CAD build for the part. Positions are in the model's coordinates, mm. A direction names the side the tool comes from. Give positions to 0.01 mm unless a question says otherwise; leave off trailing zeros. Order: outer loops, then holes, each group sorted by start corner. A loop starts at its lowest first (then second) coordinate and runs counter-clockwise, first axis right, second up. Notation, with made-up numbers: (37, 22.5) -> (79, 22.5) arc R23 ccw to (79, 34.5) -> close; hole circle Ø1 at (88, 28.5). An arc over 180 degrees is marked (long way). Use one line per item in the form item = value. Start each with the question number.
1) Mould opens along X. For faces 4 (the face through (-16.345, 29.521, 1.521)), 5 (the face through (-0.47, 58.4, -4.14)), 6 (the face through (-18.93, -43.5, 1.48)) say: pulls with the +X half, pulls with the -X half, needs draft (parallel to the pull), parting line crosses it, or undercut.
2) Probe line 1 (X direction, y = -25, z = 1.2); line 2 (Z direction, x = 15.5, y = 42); line 3 (Y direction, x = 0, z = 2.3). List the from-to ranges inside material, lowest first.
3) Cut at B-B, the plane x = -4. Give the cut face in (y, z).
4) Cut at D-D, the plane y = -14.5. Give the cut face in (x, z).
5) Tool access for faces 1 (the face through (15, 26, 2)), 2 (the face through (-20, 15, 0)), 3 (the face through (-17.5, 2, 2)): list every direction of +Z, -Z, +X, -X, +Y, -Y with a clear straight run to the whole face (end or side of a thin tool).
6) Cut at A-A, the plane y = 3. Give the cut face in (x, z).
7) Cut at C-C, the plane y = -27.5. Give the cut face in (x, z).
8) Drop flat-ended pins along their axis: P1, Ø2.5, axis at x = -14.5, z = -2.5, coming from the -Y side; P2, Ø1.5, axis at y = -29, z = 2, coming from the -X side; P3, Ø3, axis at x = -17.5, y = 30, coming from the -Z side; P4, Ø2.5, axis at x = -36, y = -40, coming from the +Z side. Give the stop position or say it passes through.
from build123d import *

# Parameters (mm, degrees)
SKETCH_1_R                  = 1.6
EXTRUDE_1_DEPTH             = 3
CUT_EXTRUDE_1_REACH         = 72.365
SKETCH_2_W                  = 30
SKETCH_2_H                  = 35
CUT_EXTRUDE_2_REACH         = 72.365
SKETCH_3_W                  = 35
SKETCH_3_H                  = 55
CUT_EXTRUDE_3_REACH         = 72.365
SKETCH_4_W                  = 25
SKETCH_4_H                  = 10
EXTRUDE_2_REACH             = 72.365
EXTRUDE_2_DIRECTION_2_REACH = 72.365
EXTRUDE_3_DEPTH             = 35
EXTRUDE_3_DEPTH_BACK        = 35
FILLET_1_R                  = 5
CUT_EXTRUDE_5_REACH         = 99.66
SKETCH_8_W                  = 70
SKETCH_8_H                  = 5
CUT_EXTRUDE_4_REACH         = 99.66
CUT_EXTRUDE_6_REACH         = 101.977
SKETCH_9_W                  = 30
SKETCH_9_H                  = 3
FILLET_2_R                  = 5
CUT_EXTRUDE_7_REACH         = 76.866
SKETCH_10_R                 = 1.25
SKETCH_11_R                 = 5
SKETCH_11_R_2               = 1.25
EXTRUDE_4_DEPTH             = 3


with BuildPart() as part:
    # 草图1 → 凸台-拉伸1 (new body)
    with BuildSketch(Plane.XY):
        Polygon((-30, 56), (30, 56), (42.5, -45), (-42.5, -45), align=None)
        with Locations((-32.5, 0)):
            Circle(SKETCH_1_R, mode=Mode.SUBTRACT)
        with Locations((32.5, 0)):
            Circle(SKETCH_1_R, mode=Mode.SUBTRACT)
        with Locations((-22, 44.5)):
            Circle(SKETCH_1_R, mode=Mode.SUBTRACT)
        with Locations(Location((22, 44.5, 0), (0, 0, 180))):
            Circle(SKETCH_1_R, mode=Mode.SUBTRACT)
        with Locations((0, 46)):
            Circle(SKETCH_1_R, mode=Mode.SUBTRACT)
        with Locations((-36, -40)):
            Circle(SKETCH_1_R, mode=Mode.SUBTRACT)
    extrude(amount=EXTRUDE_1_DEPTH)

    # 草图2 → 切除-拉伸1 (cut, up to next)
    with BuildSketch(Plane.XY.offset(3), mode=Mode.PRIVATE) as cut_extrude_1_sk1:
        with Locations((27.5, -27.5)):
            Rectangle(SKETCH_2_W, SKETCH_2_H)
    cut_extrude_1_tool1 = extrude(cut_extrude_1_sk1.sketch, amount=-CUT_EXTRUDE_1_REACH, mode=Mode.PRIVATE) & part.part
    add(cut_extrude_1_tool1.solids().sort_by_distance((27.5, -27.5, 3))[0], mode=Mode.SUBTRACT)

    # 草图3 → 切除-拉伸2 (cut, up to next)
    with BuildSketch(Plane.XY.offset(3), mode=Mode.PRIVATE) as cut_extrude_2_sk1:
        with Locations((0, -1.5)):
            Rectangle(SKETCH_3_W, SKETCH_3_H)
    cut_extrude_2_tool1 = extrude(cut_extrude_2_sk1.sketch, amount=-CUT_EXTRUDE_2_REACH, mode=Mode.PRIVATE) & part.part
    add(cut_extrude_2_tool1.solids().sort_by_distance((0, -1.5, 3))[0], mode=Mode.SUBTRACT)

    # 草图4 → 切除-拉伸3 (cut, up to next)
    with BuildSketch(Plane.XY.offset(3), mode=Mode.PRIVATE) as cut_extrude_3_sk1:
        with Locations((-5, 31)):
            Rectangle(SKETCH_4_W, SKETCH_4_H)
    cut_extrude_3_tool1 = extrude(cut_extrude_3_sk1.sketch, amount=-CUT_EXTRUDE_3_REACH, mode=Mode.PRIVATE) & part.part
    add(cut_extrude_3_tool1.solids().sort_by_distance((-5, 31, 3))[0], mode=Mode.SUBTRACT)

    # 凸台-拉伸2: up to this plane
    extrude_2_end = Plane(origin=(30, 56, 3), z_dir=(-0.9924283093332451, -0.12282528580856998, 0))
    # 草图5 → 凸台-拉伸2 (add, up to the surface)
    with BuildSketch(Plane(origin=(0, 0, 0), x_dir=(0, 0, -1), z_dir=(1, 0, 0)), mode=Mode.PRIVATE) as extrude_2_sk1:
        Polygon((0, 56), (-3, 58.517298894), (-3, 56), align=None)
    extrude_2_tool1 = split(extrude(extrude_2_sk1.sketch, amount=EXTRUDE_2_REACH, mode=Mode.PRIVATE), bisect_by=extrude_2_end, keep=Keep.BOTH, mode=Mode.PRIVATE)
    add(extrude_2_tool1.solids().sort_by_distance((0, 56.8391, 2))[0])

    # 凸台-拉伸2 direction 2: up to this plane
    extrude_2_direction_2_end = Plane(origin=(-30, 56, 3), z_dir=(0.9924283093332451, -0.12282528580856998, 0))
    # 草图5 → 凸台-拉伸2 direction 2 (add, up to the surface)
    with BuildSketch(Plane(origin=(0, 0, 0), x_dir=(0, 0, -1), z_dir=(1, 0, 0)), mode=Mode.PRIVATE) as extrude_2_direction_2_sk1:
        Polygon((0, 56), (-3, 58.517298894), (-3, 56), align=None)
    extrude_2_direction_2_tool1 = split(extrude(extrude_2_direction_2_sk1.sketch, amount=-EXTRUDE_2_DIRECTION_2_REACH, mode=Mode.PRIVATE), bisect_by=extrude_2_direction_2_end, keep=Keep.BOTH, mode=Mode.PRIVATE)
    add(extrude_2_direction_2_tool1.solids().sort_by_distance((0, 56.8391, 2))[0])

    # 草图6 → 凸台-拉伸3 (add, two sides: drawn at the far end of the back side and taken through both)
    with BuildSketch(Plane(origin=(0, 0, 0), x_dir=(0, 0, -1), z_dir=(1, 0, 0)).offset(-EXTRUDE_3_DEPTH_BACK)):
        Polygon((-3, 58.517298894), (-3, 64.391631696), (7.552988675, 55.536622791), (4.660444431, 52.089422797), (-3, 52.089422797), align=None)
    extrude(amount=EXTRUDE_3_DEPTH + EXTRUDE_3_DEPTH_BACK)

    # 圆角1
    # the kernel refuses this fillet: 5 mm, written as the material it adds along each edge
    with BuildSketch(Plane(origin=(-30.483982327, 52.089422797, 3), x_dir=(-1, 0, 0), z_dir=(0, 0, -1)), Plane(origin=(30.483982327, 52.089422797, 0), x_dir=(1, 0, 0), z_dir=(0, 0, 1))) as fillet_1_piece_1:
        with BuildLine():
            CenterArc((5.641090005, -4.871777114), FILLET_1_R, 103.003728842, 84.05145722)
            Line((0.678948458, -5.485903543), (0.579705627, -5.498186072))
            Line((0.579705627, -5.498186072), (-0.099242831, -0.012282529))
            Line((-0.099242831, -0.012282529), (0, 0.1))
            ThreePointArc((0, 0.1), (2.258008836, 0.1), (4.493516226, 0.097435542))
            Line((4.493516226, 0.097435542), (4.516017673, 0))
        make_face()
    extrude(amount=3)

    # 草图8 → 切除-拉伸5 (cut, up to next)
    with BuildSketch(Plane(origin=(0, 36.309348969, -30.467161328), x_dir=(1, 0, 0), z_dir=(0, 0.7660444431189815, -0.6427876096865354)), mode=Mode.PRIVATE) as cut_extrude_5_sk1:
        with Locations((0, -41.188276351)):
            Rectangle(SKETCH_8_W, SKETCH_8_H)
    cut_extrude_5_tool1 = extrude(cut_extrude_5_sk1.sketch, amount=-CUT_EXTRUDE_5_REACH, mode=Mode.PRIVATE) & part.part
    add(cut_extrude_5_tool1.solids().sort_by_distance((0, 62.784663, 1.084889))[0], mode=Mode.SUBTRACT)

    # 草图7 → 切除-拉伸4 (cut, up to next)
    with BuildSketch(Plane(origin=(0, 36.309348969, -30.467161328), x_dir=(1, 0, 0), z_dir=(0, 0.7660444431189815, -0.6427876096865354)), mode=Mode.PRIVATE) as cut_extrude_4_sk1:
        with BuildLine():
            Line((-35, -23.688276351), (-35, -38.688276351))
            Line((-35, -38.688276351), (-20, -38.688276351))
            ThreePointArc((-20, -38.688276351), (-30.606601718, -34.294878069), (-35, -23.688276351))
        make_face()
    cut_extrude_4_tool1 = extrude(cut_extrude_4_sk1.sketch, amount=-CUT_EXTRUDE_4_REACH, mode=Mode.PRIVATE) & part.part
    # 草图7 → 切除-拉伸4 (cut, up to next)
    with BuildSketch(Plane(origin=(0, 36.309348969, -30.467161328), x_dir=(1, 0, 0), z_dir=(0, 0.7660444431189815, -0.6427876096865354)), mode=Mode.PRIVATE) as cut_extrude_4_sk2:
        with BuildLine():
            Line((35, -38.688276351), (20, -38.688276351))
            ThreePointArc((20, -38.688276351), (30.606601718, -34.294878069), (35, -23.688276351))
            Line((35, -23.688276351), (35, -38.688276351))
        make_face()
    cut_extrude_4_tool2 = extrude(cut_extrude_4_sk2.sketch, amount=-CUT_EXTRUDE_4_REACH, mode=Mode.PRIVATE) & part.part
    add(cut_extrude_4_tool1.solids().sort_by_distance((-31.649481, 59.024021, -3.396869))[0], mode=Mode.SUBTRACT)
    add(cut_extrude_4_tool2.solids().sort_by_distance((31.649481, 59.024021, -3.396869))[0], mode=Mode.SUBTRACT)

    # 草图9 → 切除-拉伸6 (cut, up to next)
    with BuildSketch(Plane(origin=(0, -29, 0), x_dir=(1, 0, 0), z_dir=(0, 1, 0)), mode=Mode.PRIVATE) as cut_extrude_6_sk1:
        with Locations((-2.5, -1.5)):
            Rectangle(SKETCH_9_W, SKETCH_9_H)
    cut_extrude_6_tool1 = extrude(cut_extrude_6_sk1.sketch, amount=-CUT_EXTRUDE_6_REACH, mode=Mode.PRIVATE) & part.part
    add(cut_extrude_6_tool1.solids().sort_by_distance((-2.5, -29, 1.5))[0], mode=Mode.SUBTRACT)

    # 圆角2
    fillet_2_edges = [part.edges().sort_by_distance(p)[0] for p in [
        (-17.5, -45, 1.5),
        (38.168316832, -10, 1.5),
        (17.5, -10, 1.5),
        (7.5, 26, 1.5),
        (-42.5, -45, 1.5),
    ]]
    fillet(fillet_2_edges, radius=FILLET_2_R)

    # 草图10 → 切除-拉伸7 (cut, up to next)
    with BuildSketch(Plane.XY.offset(3), mode=Mode.PRIVATE) as cut_extrude_7_sk1:
        with Locations((17.5, 30)):
            Circle(SKETCH_10_R)
    cut_extrude_7_tool1 = extrude(cut_extrude_7_sk1.sketch, amount=-CUT_EXTRUDE_7_REACH, mode=Mode.PRIVATE) & part.part
    # 草图10 → 切除-拉伸7 (cut, up to next)
    with BuildSketch(Plane.XY.offset(3), mode=Mode.PRIVATE) as cut_extrude_7_sk2:
        with Locations((-17.5, 30)):
            Circle(SKETCH_10_R)
    cut_extrude_7_tool2 = extrude(cut_extrude_7_sk2.sketch, amount=-CUT_EXTRUDE_7_REACH, mode=Mode.PRIVATE) & part.part
    # 草图10 → 切除-拉伸7 (cut, up to next)
    with BuildSketch(Plane.XY.offset(3), mode=Mode.PRIVATE) as cut_extrude_7_sk3:
        with Locations((-17.5, -25)):
            Circle(SKETCH_10_R)
    cut_extrude_7_tool3 = extrude(cut_extrude_7_sk3.sketch, amount=-CUT_EXTRUDE_7_REACH, mode=Mode.PRIVATE) & part.part
    add(cut_extrude_7_tool1.solids().sort_by_distance((17.5, 30, 3))[0], mode=Mode.SUBTRACT)
    add(cut_extrude_7_tool2.solids().sort_by_distance((-17.5, 30, 3))[0], mode=Mode.SUBTRACT)
    add(cut_extrude_7_tool3.solids().sort_by_distance((-17.5, -25, 3))[0], mode=Mode.SUBTRACT)

    # 草图11 → 凸台-拉伸4 (add)
    # profile 1 of 2: a face of its own
    with BuildSketch(Plane.XY.offset(3)):
        with Locations((-17.5, -25)):
            Circle(SKETCH_11_R)
        with Locations((-17.5, -25)):
            Circle(SKETCH_11_R_2, mode=Mode.SUBTRACT)
    # profile 2 of 2: a face of its own
    with BuildSketch(Plane.XY.offset(3)):
        with BuildLine():
            Line((-12.5, 30), (-12.5, 36))
            Line((-12.5, 36), (-17.5, 36))
            Line((-17.5, 36), (-17.5, 35))
            ThreePointArc((-17.5, 35), (-21.035533906, 26.464466094), (-12.5, 30))
        make_face()
        with Locations((-17.5, 30)):
            Circle(SKETCH_11_R_2, mode=Mode.SUBTRACT)
    extrude(amount=-EXTRUDE_4_DEPTH)


solid = part.part
Result:
q1.face_4 = undercut
q1.face_5 = needs draft
q1.face_6 = pulls with the +X half
q2.line_1 = -40.02 to -18.75, -16.25 to -12.5
q2.line_2 = 0 to 3
q2.line_3 = 36 to 44.4, 47.6 to 57.45
q3.outline = (36, 0) -> (52.09, 0) -> (52.09, -4.66) -> (55.54, -7.55) -> (61.18, -0.83) -> (56.61, 3) -> (36, 3) -> close
q4.outline = (-38.73, 0) -> (-17.5, 0) -> (-17.5, 3) -> (-38.73, 3) -> close
q5.face_1 = +Z, -Z, -Y
q5.face_2 = -Z, +X, -X, -Y
q5.face_3 = +Z, -Z
q6.outline = (-36.56, 0) -> (-17.5, 0) -> (-17.5, 3) -> (-36.56, 3) -> close; (17.5, 0) -> (36.56, 0) -> (36.56, 3) -> (17.5, 3) -> close
q7.outline = (-40.33, 0) -> (-13.17, 0) -> (-13.17, 3) -> (-40.33, 3) -> close
q8.P1 = 52.09
q8.P2 = -40.61
q8.P3 = 0
q8.P4 = through
